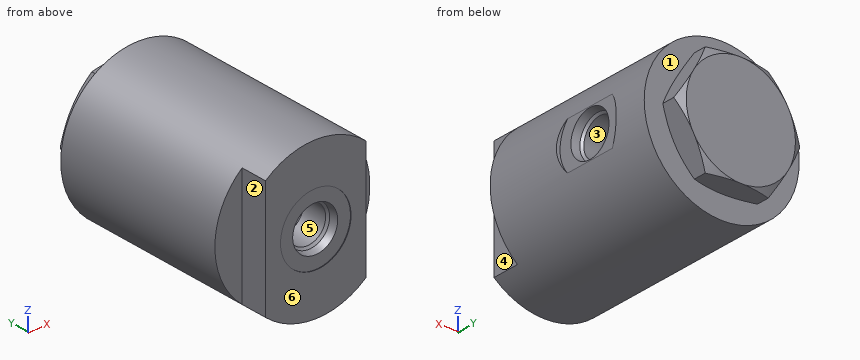
```python
from build123d import *

# Parameters (mm, degrees)
SKETCH1_R          = 27.051
EXTRUDE1_DEPTH     = 73.152
CUT_EXTRUDE1_DEPTH = 9.652
EXTRUDE2_DEPTH     = 7.874
SKETCH7_W          = 15.875
SKETCH7_H          = 60.325


with BuildPart() as part:
    # Sketch1 → Extrude1 (new body)
    with BuildSketch(Plane(origin=(0, 0, 0), x_dir=(1, 0, 0), z_dir=(0, 1, 0))):
        with Locations(Location((0, 0, 0), (0, 0, 270))):  # turned: the seam where the file's is
            Circle(SKETCH1_R)
    extrude(amount=EXTRUDE1_DEPTH)

    # Sketch2 → Cut-Extrude1 (cut)
    with BuildSketch(Plane.XZ):
        with BuildLine():
            Line((17.526, 20.605725539), (17.526, -20.605725539))
            ThreePointArc((17.526, -20.605725539), (27.051, 0), (17.526, 20.605725539))
        make_face()
        with BuildLine():
            Line((-17.526, -20.605725539), (-17.526, 20.605725539))
            ThreePointArc((-17.526, 20.605725539), (-27.051, 0), (-17.526, -20.605725539))
        make_face()
    extrude(amount=-CUT_EXTRUDE1_DEPTH, mode=Mode.SUBTRACT)

    # S2D0007 → Cut-Revolve1 (revolve, cut)
    with BuildSketch(Plane(origin=(27.051, 49.276, 0), x_dir=(0, -1, 0), z_dir=(0, 0, 1)), mode=Mode.PRIVATE) as cut_revolve1_sk:
        Polygon((0, 0), (12.319, 0), (12.319, -1.27), (7.85495, -1.27), (7.290761118, -3.9243), (6.5405, -4.674561118), (6.5405, -16.7386), (0, -20.668528879), align=None)
    revolve(cut_revolve1_sk.sketch.rotate(Axis((-4.448190263, 49.276, 0), (1, 0, 0)), 270), axis=Axis((-4.448190263, 49.276, 0), (1, 0, 0)), mode=Mode.SUBTRACT)  # turned: the seam where the file's is

    # Sketch4 → Cut-Revolve2 (revolve, cut)
    with BuildSketch(Plane(origin=(0, 0, 0), x_dir=(-1, 0, 0), z_dir=(0, 0, 1)), mode=Mode.PRIVATE) as cut_revolve2_sk:
        Polygon((0, 0), (12.319, 0), (12.319, -0.254), (7.85495, -0.254), (7.290761118, -2.9083), (6.5405, -3.658561118), (6.5405, -15.7226), (0, -19.652528879), align=None)
    revolve(cut_revolve2_sk.sketch.rotate(Axis((0, 25.899297965, 0), (0, -1, 0)), 270), axis=Axis((0, 25.899297965, 0), (0, -1, 0)), mode=Mode.SUBTRACT)  # turned: the seam where the file's is

    # Sketch5 → Extrude2 (add)
    with BuildSketch(Plane(origin=(0, 73.152, 0), x_dir=(-1, 0, 0), z_dir=(0, 1, 0))):
        Polygon((21.997045256, 0), (10.998522628, 19.05), (-10.998522628, 19.05), (-21.997045256, 0), (-10.998522628, -19.05), (10.998522628, -19.05), align=None)
    extrude(amount=EXTRUDE2_DEPTH)

    # Sketch6 → Cut-Revolve3 (revolve, cut)
    with BuildSketch(Plane(origin=(0, 0, 0), x_dir=(0, 0, -1), z_dir=(1, 0, 0)), mode=Mode.PRIVATE) as cut_revolve3_sk:
        Polygon((19.05, 81.026), (25.869084029, 77.089), (19.05, 73.152), (31.75, 73.152), (31.75, 81.026), align=None)
    revolve(cut_revolve3_sk.sketch.rotate(Axis((0, 72.7583, 0), (0, 1, 0)), 180), axis=Axis((0, 72.7583, 0), (0, 1, 0)), mode=Mode.SUBTRACT)  # turned: the seam where the file's is

    # Sketch7 → Cut-Revolve4 (revolve, cut)
    with BuildSketch(Plane.XY, mode=Mode.PRIVATE) as cut_revolve4_sk:
        with Locations((-7.9375, 42.9895)):
            Rectangle(SKETCH7_W, SKETCH7_H)
    revolve(cut_revolve4_sk.sketch.rotate(Axis((0, 0, 0), (0, 1, 0)), 90), axis=Axis((0, 0, 0), (0, 1, 0)), mode=Mode.SUBTRACT)  # turned: the seam where the file's is


solid = part.part
```
Design review of the part built by this model. Coordinates are the model's own, in mm. Face numbers are marked on the shaded views. A direction names the side the tool comes from. Give positions to 0.01 mm unless a question says otherwise; leave off trailing zeros. Loops run counter-clockwise (first coordinate to the right, second up) from the corner with the lowest first, then second, coordinate; pieces in that order, holes last. Notation, with made-up numbers: (75.25, 51.25) -> (126.25, 51.25) arc R28 cw to (126.25, 78.25) -> close; hole circle Ø1 at (27, -2.5). An arc over 180 degrees is marked (long way). Write each question's results on one line, items separated by ' | '.
Q1. Take a section at A-A, the plane y = 38.5. Write out the cut boundary in (x, z) (3 decimals).
Reply:
outline: (25.781, -5.97) -> (25.781, 5.97) -> (26.384, 5.97) arc R27.051 ccw (long way) to (26.384, -5.97) -> close; hole circle Ø31.75 at (0, 0)
Q2. Wall thickness on L1, parallel to X at y = 0.1, z = 0; L2, parallel to X at y = 8, z = 0; L3, parallel to Y at x = 0.5, z = 15.5: over which ranges is each line inside the solid? List them lowest first.
Reply:
L1: x = -17.53 to -12.32, 12.32 to 17.53 | L2: x = -17.53 to -6.54, 6.54 to 17.53 | L3: y = 0 to 12.83, 73.15 to 81.03
Q3. The part is to be moulded in two halves that separate along X. For the marked faces 4, 5 and 6, say which applies: +X half, -X half, draft (parallel to the pull), parting line (faces both ways), or undercut.
Reply:
face 4: +X half | face 5: undercut | face 6: draft
Q4. Take a section at B-B, the plane y = 5. Write out the cut boundary in (x, z), plus the area to 3 significant figures.
Reply:
outline: (-17.53, -20.61) arc R27.05 ccw to (17.53, -20.61) -> (17.53, 20.61) arc R27.05 ccw to (-17.53, 20.61) -> close; hole circle Ø13.08 at (0, 0) | area: 1,620 mm²
Q5. Take a section at C-C, the plane z = 22. Write out the cut boundary in (x, y), plus the area to 3 significant figures.
Reply:
outline: (-15.74, 0) -> (15.74, 0) -> (15.74, 73.15) -> (-15.74, 73.15) -> close | area: 2,300 mm²
Q6. Take a section at D-D, the plane y = 27. Write out the cut boundary in (x, z) (3 decimals).
Reply:
outline: circle Ø54.102 at (0, 0); hole circle Ø31.75 at (0, 0)
Q7. For pin 1 Ø4 at (y, z) = (41, -13.5) entering from -X; pin 2 Ø5 at (x, z) = (22, -9.5) entering from -Y; pin 3 Ø1 at (y, z) = (15, 5.5) entering from +X, all flat-tipped, find the tip position at first contact; note any pin that passes through.
Reply:
pin 1: stops at x = -24.48 | pin 2: stops at y = 9.65 | pin 3: stops at x = 26.58
Q8. Machinability: for the marked faces 1, 2 and 3, which of the approach directions +Z, -Z, +X, -X, +Y, -Y give a long, thin tool a straight path to every point of the face, cutting with its end or side? Answer none if there is none.
Reply:
face 1: none | face 2: +Z, -Z, -X, -Y | face 3: +X
